from build123d import *

# Parameters (mm, degrees)
SKETCH1_W             = 25.4
SKETCH1_H             = 50.8
SKETCH1_W_2           = 19.05
SKETCH1_H_2           = 44.45
BOSS_EXTRUDE1_DEPTH   = 225.02495
F_8_32_TAPPED_HOLE1_D = 3.4544
CUT_EXTRUDE1_DEPTH    = 228.873974211
FILLET1_R             = 3.175


with BuildPart() as part:
    # Sketch1 → Boss-Extrude1 (new, symmetric)
    with BuildSketch(Plane(origin=(0, 0, 0), x_dir=(0, 0, -1), z_dir=(1, 0, 0))):
        Rectangle(SKETCH1_W, SKETCH1_H)
        Rectangle(SKETCH1_W_2, SKETCH1_H_2, mode=Mode.SUBTRACT)
    extrude(amount=BOSS_EXTRUDE1_DEPTH, both=True)

    # #8-32 Tapped Hole1 (through all)
    with Locations(Plane.XY.offset(12.7)):
        with Locations((-212.32495, 12.7), (-212.32495, -12.7), (-199.62495, 0), (212.32495, 12.7), (199.62495, 0), (212.32495, -12.7)):
            Hole(F_8_32_TAPPED_HOLE1_D / 2)

    # Sketch4 → Cut-Extrude1 (cut, through all)
    with BuildSketch(Plane.XY.offset(12.7)):
        Polygon((-186.92495, 15.875), (-186.92495, -15.875), (-153.930599661, 15.875), align=None)
        Polygon((-140.1937125, 15.875), (-173.188062839, -15.875), (-107.199362161, -15.875), align=None)
        Polygon((-126.456825339, 15.875), (-93.462475, -15.875), (-60.468124661, 15.875), align=None)
        Polygon((-46.7312375, 15.875), (-79.725587839, -15.875), (-13.736887161, -15.875), align=None)
        Polygon((-32.994350339, 15.875), (0, -15.875), (32.994350339, 15.875), align=None)
        Polygon((13.736887161, -15.875), (46.7312375, 15.875), (79.725587839, -15.875), align=None)
        Polygon((60.468124661, 15.875), (93.462475, -15.875), (126.456825339, 15.875), align=None)
        Polygon((107.199362161, -15.875), (140.1937125, 15.875), (173.188062839, -15.875), align=None)
        Polygon((186.92495, 15.875), (186.92495, -15.875), (153.930599661, 15.875), align=None)
    extrude(amount=-CUT_EXTRUDE1_DEPTH, mode=Mode.SUBTRACT)

    # Fillet1
    fillet1_edges = [part.edges().sort_by_distance(p)[0] for p in [
        (-186.92495, 15.875, -11.1125),
        (-153.930599661, 15.875, -11.1125),
        (-186.92495, -15.875, -11.1125),
        (-186.92495, 15.875, 11.1125),
        (-153.930599661, 15.875, 11.1125),
        (-186.92495, -15.875, 11.1125),
        (-140.1937125, 15.875, -11.1125),
        (-107.199362161, -15.875, -11.1125),
        (-173.188062839, -15.875, -11.1125),
        (-140.1937125, 15.875, 11.1125),
        (-107.199362161, -15.875, 11.1125),
        (-173.188062839, -15.875, 11.1125),
        (-126.456825339, 15.875, -11.1125),
        (-60.468124661, 15.875, -11.1125),
        (-93.462475, -15.875, -11.1125),
        (-126.456825339, 15.875, 11.1125),
        (-60.468124661, 15.875, 11.1125),
        (-93.462475, -15.875, 11.1125),
        (-46.7312375, 15.875, -11.1125),
        (-13.736887161, -15.875, -11.1125),
        (-79.725587839, -15.875, -11.1125),
        (-46.7312375, 15.875, 11.1125),
        (-13.736887161, -15.875, 11.1125),
        (-79.725587839, -15.875, 11.1125),
        (-32.994350339, 15.875, -11.1125),
        (32.994350339, 15.875, -11.1125),
        (0, -15.875, -11.1125),
        (-32.994350339, 15.875, 11.1125),
        (32.994350339, 15.875, 11.1125),
        (0, -15.875, 11.1125),
        (79.725587839, -15.875, -11.1125),
        (13.736887161, -15.875, -11.1125),
        (46.7312375, 15.875, -11.1125),
        (79.725587839, -15.875, 11.1125),
        (13.736887161, -15.875, 11.1125),
        (46.7312375, 15.875, 11.1125),
        (60.468124661, 15.875, -11.1125),
        (126.456825339, 15.875, -11.1125),
        (93.462475, -15.875, -11.1125),
        (60.468124661, 15.875, 11.1125),
        (126.456825339, 15.875, 11.1125),
        (93.462475, -15.875, 11.1125),
        (173.188062839, -15.875, -11.1125),
        (107.199362161, -15.875, -11.1125),
        (140.1937125, 15.875, -11.1125),
        (173.188062839, -15.875, 11.1125),
        (107.199362161, -15.875, 11.1125),
        (140.1937125, 15.875, 11.1125),
        (153.930599661, 15.875, -11.1125),
        (186.92495, 15.875, -11.1125),
        (186.92495, -15.875, -11.1125),
        (153.930599661, 15.875, 11.1125),
        (186.92495, 15.875, 11.1125),
        (186.92495, -15.875, 11.1125),
    ]]
    fillet(fillet1_edges, radius=FILLET1_R)


solid = part.part
Could you check a few things on this model? Use its own coordinates, in mm. A direction names the side the tool comes from. Round coordinates to 2 decimals unless told otherwise and drop trailing zeros. Write each loop counter-clockwise with the first axis right and the second up, starting at its lowest first coordinate (ties: lowest second). Pieces come first, ordered by that corner, then holes. Notation, with made-up numbers: (-12.5, -7) -> (16.5, -7) arc R17 ccw to (16.5, 13) -> close; hole circle Ø5 at (85.25, 68). An arc over 180 degrees is marked (long way). Use a Markdown table: item, result.
1. We'd pull the mould along Z, two halves only. Please class faces 1 (the face through (3, 22.225, 0)), 2 (the face through (3, -22.225, 0)), 3 (the face through (3, 17, 12.7)), 4 (the face through (-14.94, -1.5, 11.13)): +Z half, -Z half, draft (parallel to the pull), parting line (faces both ways), or undercut.
Answer key:
| item | result |
|---|---|
| face 1 | undercut |
| face 2 | undercut |
| face 3 | +Z half |
| face 4 | draft |
2. If we section it at C-C (x = 86.5): List the corners of the cut face in (y, z) for me (3 decimals), then the cut area to 3 significant figures.
Answer key:
| item | result |
|---|---|
| outline | (-25.4, -12.7) -> (-9.175, -12.7) -> (-9.175, -9.525) -> (-22.225, -9.525) -> (-22.225, 9.525) -> (-9.175, 9.525) -> (-9.175, 12.7) -> (-25.4, 12.7) -> close; (15.875, -12.7) -> (25.4, -12.7) -> (25.4, 12.7) -> (15.875, 12.7) -> (15.875, 9.525) -> (22.225, 9.525) -> (22.225, -9.525) -> (15.875, -9.525) -> close |
| area | 284 mm^2 |
3. If we section it at B-B (x = 132): List the corners of the cut face in (y, z) for me (3 decimals), then the cut area to 3 significant figures.
Answer key:
| item | result |
|---|---|
| outline | (-25.4, -12.7) -> (-15.875, -12.7) -> (-15.875, -9.525) -> (-22.225, -9.525) -> (-22.225, 9.525) -> (-15.875, 9.525) -> (-15.875, 12.7) -> (-25.4, 12.7) -> close; (7.99, -12.7) -> (25.4, -12.7) -> (25.4, 12.7) -> (7.99, 12.7) -> (7.99, 9.525) -> (22.225, 9.525) -> (22.225, -9.525) -> (7.99, -9.525) -> close |
| area | 292 mm^2 |
4. Please list where these lines run through material, in increasing order: probe 1 along Y at (x, z) = (-62.5, 7) (3 decimals); probe 2 along Z at (x, y) = (-36, 14.5) (3 decimals); probe 3 along Y at (x, z) = (-114, 11.75) (3 decimals).
Answer key:
| item | result |
|---|---|
| probe 1 | y = -25.4 to -22.225, 22.225 to 25.4 |
| probe 2 | z = -12.7 to -9.525, 9.525 to 12.7 |
| probe 3 | y = -25.4 to -15.686, -9.331 to 3.888, 15.875 to 25.4 |
5. If we section it at A-A (z = 3.75): List the corners of the cut face in (x, y) for me (3 decimals), then the cut area to 3 significant figures.
Answer key:
| item | result |
|---|---|
| outline | (-225.025, -25.4) -> (225.025, -25.4) -> (225.025, -22.225) -> (-225.025, -22.225) -> close; (-225.025, 22.225) -> (225.025, 22.225) -> (225.025, 25.4) -> (-225.025, 25.4) -> close |
| area | 2,860 mm^2 |
6. Which directions (+Z, -Z, +X, -X, +Y, -Y) give clear straight access to the entire face, cutting with the end or side of a thin tool? Please do faces 5 (the face through (3, 25.4, 0)), 6 (the face through (3, -15, -9.525)), 7 (the face through (154.78, 1.84, 11.13)).
Answer key:
| item | result |
|---|---|
| face 5 | +Z, -Z, +X, -X, +Y |
| face 6 | +X, -X |
| face 7 | +Z, -Z |
